Autodesk Inventor part; units mm, degrees
ref_plane "YZ Plane" through (0, 0, 0) normal (1, 0, 0) x (0, 1, 0)
ref_plane "XZ Plane" through (0, 0, 0) normal (0, 1, 0) x (-1, 0, 0)
ref_plane "XY Plane" through (0, 0, 0) normal (0, 0, 1) x (1, 0, 0)
ref_plane "Work Plane2" through (0, 147.11, 157.65) normal (0, 0, 1) x (1, 0, 0)
sketch "Sketch2" plane through (0, 147.11, 157.65) normal (0, 0, 1) x (1, 0, 0)
  arc A0 (61.9417, -3.175) -> (58.7667, 0) centre (58.7667, -3.175) ccw
  line L0 (58.7667, 0) -> (55.1167, 0)
  arc A1 (51.9417, 3.175) -> (55.1167, 0) centre (55.1167, 3.175) ccw
  arc A2 (51.9417, 3.937) -> (48.7667, 7.112) centre (48.7667, 3.937) ccw
  line L1 (48.7667, 7.112) -> (-48.7667, 7.112)
  arc A3 (-48.7667, 7.112) -> (-51.9417, 3.937) centre (-48.7667, 3.937) ccw
  arc A4 (-55.1167, 0) -> (-51.9417, 3.175) centre (-55.1167, 3.175) ccw
  line L2 (-55.1167, 0) -> (-58.7667, 0)
  arc A5 (-58.7667, 0) -> (-61.9417, -3.175) centre (-58.7667, -3.175) ccw
  line L3 (-61.9417, -3.175) -> (-61.9417, -14.325)
  arc A6 (-61.9417, -14.325) -> (-58.7667, -17.5) centre (-58.7667, -14.325) ccw
  line L4 (-58.7667, -17.5) -> (58.7667, -17.5)
  arc A7 (58.7667, -17.5) -> (61.9417, -14.325) centre (58.7667, -14.325) ccw
  line L5 (61.9417, -14.325) -> (61.9417, -3.175)
  arc A8 (-44.4178, 0) -> (-42.1518, 0) centre (-43.2848, 0) ccw
  line L6 (-44.4178, 0) -> (-44.4178, 5)
  arc A9 (-42.1518, 5) -> (-44.4178, 5) centre (-43.2848, 5) ccw
  line L7 (-42.1518, 5) -> (-42.1518, 0)
  circle A10 centre (56.9417, -12.5) radius 1.524
  circle A11 centre (-56.9417, -3.75) radius 1.524
  circle A12 centre (56.9417, -3.75) radius 1.524
  circle A13 centre (-43.2848, -3.75) radius 1.27
  circle A14 centre (-25.9709, -3.75) radius 1.27
  circle A15 centre (-8.657, -3.75) radius 1.27
  circle A16 centre (8.657, -3.75) radius 1.27
  circle A17 centre (25.9709, -3.75) radius 1.27
  circle A18 centre (43.2848, -3.75) radius 1.27
  circle A19 centre (-56.9417, -12.5) radius 1.524
  arc A20 (-27.1039, 0) -> (-24.8379, 0) centre (-25.9709, 0) ccw
  line L8 (-27.1039, 0) -> (-27.1039, 5)
  arc A21 (-24.8379, 5) -> (-27.1039, 5) centre (-25.9709, 5) ccw
  line L9 (-24.8379, 5) -> (-24.8379, 0)
  arc A22 (-9.79, 0) -> (-7.524, 0) centre (-8.657, 0) ccw
  line L10 (-9.79, 0) -> (-9.79, 5)
  arc A23 (-7.524, 5) -> (-9.79, 5) centre (-8.657, 5) ccw
  line L11 (-7.524, 5) -> (-7.524, 0)
  arc A24 (7.524, 0) -> (9.79, 0) centre (8.657, 0) ccw
  line L12 (7.524, 0) -> (7.524, 5)
  arc A25 (9.79, 5) -> (7.524, 5) centre (8.657, 5) ccw
  line L13 (9.79, 5) -> (9.79, 0)
  arc A26 (24.8379, 0) -> (27.1039, 0) centre (25.9709, 0) ccw
  line L14 (24.8379, 0) -> (24.8379, 5)
  arc A27 (27.1039, 5) -> (24.8379, 5) centre (25.9709, 5) ccw
  line L15 (27.1039, 5) -> (27.1039, 0)
  arc A28 (42.1518, 0) -> (44.4178, 0) centre (43.2848, 0) ccw
  line L16 (42.1518, 0) -> (42.1518, 5)
  arc A29 (44.4178, 5) -> (42.1518, 5) centre (43.2848, 5) ccw
  line L17 (44.4178, 5) -> (44.4178, 0)
  line L18 (-55.1167, 0) -> (55.1167, 0)
  circle A30 centre (-43.2848, -3.75) radius 1.778
  circle A31 centre (-25.9709, -3.75) radius 1.778
  circle A32 centre (-8.657, -3.75) radius 1.778
  circle A33 centre (8.657, -3.75) radius 1.778
  circle A34 centre (25.9709, -3.75) radius 1.778
  circle A35 centre (43.2848, -3.75) radius 1.778
  line L19 (-54.3979, -17.5) -> (54.3979, -17.5)
  line L20 (51.9417, 3.175) -> (51.9417, 3.937)
  line L21 (-51.9417, 3.937) -> (-51.9417, 3.175)
  point P0 (0, -147.11)
  point P1 (-55.1167, 3.175)
  point P2 (51.9417, 3.683)
  point P3 (-51.9417, 3.683)
  point P4 (-55.1167, 3.175)
  dimension "d0" = 3.556
  dimension "d1" = 3.556
  dimension "d2" = 3.556
  dimension "d3" = 3.556
  dimension "d4" = 3.556
  dimension "d5" = 3.556
extrude "Extrusion1" add sketch "Sketch2" along normal blind 3.175 contours L5 A7 L4 A6 L3 A5 L2 L18 A8 A20 A22 A24 A26 A28 L0 A0 | A28 L18 | A26 L18 | A24 L18 | A22 L18 | L18 A8 | A20 L18
properties part number "string_mount"
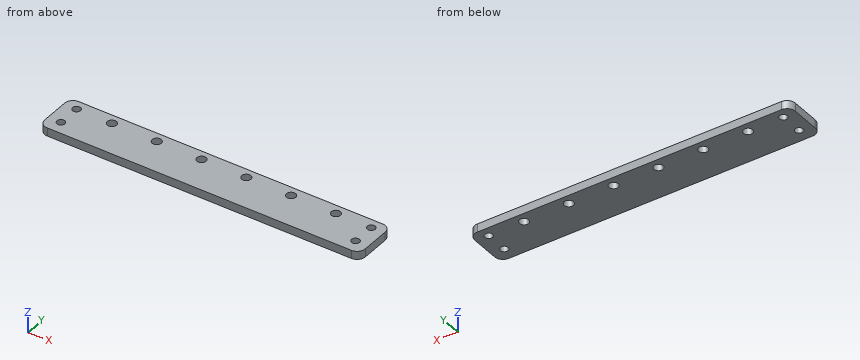
Check sheet for the modelled part. Datum: model origin and axes. Units: mm. Give positions to 0.01 mm unless a question says otherwise; leave off trailing zeros. Write each loop counter-clockwise with the first axis right and the second up, starting at its lowest first coordinate (ties: lowest second). Pieces come first, ordered by that corner, then holes. Notation, with made-up numbers: (62.5, 50.5) - (108.5, 50.5) arc R18 cw to (108.5, 83.5) - close; hole circle Ø11 at (29.5, 28). An arc over 180 degrees is marked (long way). Answer as a JSON object with one key per item and string values. Group by question number.
1) Sectioned sample at B-B (y = 134.61). Record the cut outline in (x, z) (3 decimals).
2) Thickness scan on probe 1 along Y at (x, z) = (-26, 159.15); probe 2 along Y at (x, z) = (-27, 158.8); probe 3 along X at (y, z) = (131, 158.05). Record the ranges inside material, lowest first. Write a range as from..to.
3) Sectioned sample at A-A (z = 158.55). Give the number of separate pieces and of enclosed holes in the cut face, then the cut area to 3 significant figures.
4) Depth check by flat-ended pin: P1, Ø2, axis at x = 43.28, y = 143.36, coming from the +Z side. Enter the tip coordinate at first touch or a pass-through.
Geometry results:
{
 "1": {"outline": "(-61.942, 157.65) - (-58.466, 157.65) - (-58.466, 160.825) - (-61.942, 160.825) - close; (-55.418, 157.65) - (55.418, 157.65) - (55.418, 160.825) - (-55.418, 160.825) - close; (58.466, 157.65) - (61.942, 157.65) - (61.942, 160.825) - (58.466, 160.825) - close"},
 "2": {"probe 1": "y = 129.61..141.58, 145.14..147.11", "probe 2": "y = 129.61..141.91, 144.81..147.11", "probe 3": "x = -61.39..61.39"},
 "3": {"separate pieces": "1", "enclosed holes": "10", "area": "2,070 mm^2"},
 "4": {"P1": "passes through"}
}
